Read the model definition and answer for the solid it produces. Units are mm, in the model's axes. A direction names the side the tool comes from. Give positions to 0.01 mm unless a question says otherwise; leave off trailing zeros. Loops run counter-clockwise (first coordinate to the right, second up) from the corner with the lowest first, then second, coordinate; pieces in that order, holes last. Notation, with made-up numbers: (27, 23) -> (50, 23) arc R6 ccw to (50, 27) -> close; hole circle Ø4 at (3.5, -37). An arc over 180 degrees is marked (long way). Return JSON: item names as keys, results as strings. Group by question number.
from build123d import *

# Parameters (mm, degrees)
AUFSATZ_LINEAR_AUSTRAGEN1_DEPTH = 3
SKIZZE2_R                       = 2.05
AUFSATZ_LINEAR_AUSTRAGEN2_DEPTH = 12.5
AUFSATZ_LINEAR_START            = 9.5
AUFSATZ_LINEAR_AUSTRAGEN3_DEPTH = 1.6
SCHNITT_LINEAR_AUSTRAGEN1_REACH = 19.13
SKIZZE4_R                       = 1
FASE1_SIZE                      = 0.4


with BuildPart() as part:
    # Skizze1 → Aufsatz-Linear austragen1 (new body)
    with BuildSketch(Plane.XY):
        with BuildLine():
            Line((2, 0), (2, 5))
            ThreePointArc((2, 5), (0, 7), (-2, 5))
            Line((-2, 5), (-2, 0))
            ThreePointArc((-2, 0), (0, -2), (2, 0))
        make_face()
    extrude(amount=AUFSATZ_LINEAR_AUSTRAGEN1_DEPTH)

    # Skizze2 → Aufsatz-Linear austragen2 (add)
    with BuildSketch(Plane.XY.offset(3)):
        with Locations(Location((0, 0, 0), (0, 0, 167.319616508))):
            Circle(SKIZZE2_R)
    extrude(amount=AUFSATZ_LINEAR_AUSTRAGEN2_DEPTH)

    # Skizze3 → Aufsatz-Linear austragen3 (add)
    with BuildSketch(Plane.XY.offset(3).offset(AUFSATZ_LINEAR_START)):
        with BuildLine():
            Line((-1.25, 3.5), (-1.25, 1.624807681))
            ThreePointArc((-1.25, 1.624807681), (0, 2.05), (1.25, 1.624807681))
            Line((1.25, 1.624807681), (1.25, 3.5))
            ThreePointArc((1.25, 3.5), (0, 4.75), (-1.25, 3.5))
        make_face()
    extrude(amount=AUFSATZ_LINEAR_AUSTRAGEN3_DEPTH)

    # Skizze4 → Schnitt-Linear austragen1 (cut, up to next)
    with BuildSketch(Plane.XY.offset(15.5), mode=Mode.PRIVATE) as schnitt_linear_austragen1_sk1:
        Circle(SKIZZE4_R)
    schnitt_linear_austragen1_tool1 = extrude(schnitt_linear_austragen1_sk1.sketch, amount=-SCHNITT_LINEAR_AUSTRAGEN1_REACH, mode=Mode.PRIVATE) & part.part
    add(schnitt_linear_austragen1_tool1.solids().sort_by_distance((0, 0, 15.5))[0], mode=Mode.SUBTRACT)

    # Fase1
    fase1_edges = [part.edges().sort_by_distance(p)[0] for p in [
        (2, -0.45, 15.5),
    ]]
    chamfer(fase1_edges, length=FASE1_SIZE)


solid = part.part
1. Section A-A on x = 0 is taken. Determine the outline of the cut face in (y, z).
2. Section D-D on z = 13.75 is taken. Determine the outline of the cut face in (x, y), then the cut area to 3 significant figures.
3. Section B-B on y = 2.25 is taken. Determine the outline of the cut face in (x, z), then the cut area to 3 significant figures.
4. Flat-ended cylindrical pins translate along their axes: pin 1 Ø5 at (y, z) = (0.5, 4.5) entering from -X; pin 2 Ø1.5 at (x, z) = (-0.5, 8) entering from +Y; pin 3 Ø1.8 at (y, z) = (2.5, 13.5) entering from -X; pin 4 Ø1.2 at (x, y) = (-0.5, 2.5) entering from +Z. Find the tip coordinate at first contact, or state that the pin passes through.
5. Determine the mould class of faces 1 (the flat face through (1.25, 3, 13)), 2 (the cylindrical face through (0, 7, 1)), 3 (the cylindrical face through (0, -1, 8)), 4 (the cylindrical face through (-0.19, -2.04, 8.97)) for opening direction Y: pulls with the +Y half, pulls with the -Y half, needs draft (parallel to the pull), parting line crosses it, or undercut.
6. Which of the six approach directions +Z, -Z, +X, -X, +Y, -Y give full straight-line access (tool end or side, diameter ignored) to faces 5 (the cylindrical face through (0, -2, 1)), 6 (the flat face through (-1.25, 3, 13)), 7 (the cylindrical face through (0.03, 4.75, 13.29)), 8 (the flat face through (-1, 1, 15.5))?
7. Section C-C on z = 1.25 is taken. Determine the outline of the cut face in (x, y), then the cut area to 3 significant figures.
8. Straight lines are drawn through the part: line 1 (Z direction, x = 0.05, y = 5); line 2 (X direction, y = -0.75, z = 14.75); line 3 (Z direction, x = 0.75, y = 4.25). For each, find the intervals that lie inside material, in ascending order. Write a range as from..to.
Completed:
{
 "1": {"outline": "(-2.05, 3) -> (-2, 3) -> (-2, 0) -> (-1, 0) -> (-1, 15.5) -> (-1.65, 15.5) -> (-2.05, 15.1) -> close; (1, 0) -> (7, 0) -> (7, 3) -> (2.05, 3) -> (2.05, 12.5) -> (4.75, 12.5) -> (4.75, 14.1) -> (2.05, 14.1) -> (2.05, 15.1) -> (1.65, 15.5) -> (1, 15.5) -> close"},
 "2": {"outline": "(-1.25, 1.62) arc R2.05 ccw (long way) to (1.25, 1.62) -> (1.25, 3.5) arc R1.25 ccw to (-1.25, 3.5) -> close; hole circle Ø2 at (0, 0)", "area": "16.5 mm²"},
 "3": {"outline": "(-2, 0) -> (2, 0) -> (2, 3) -> (-2, 3) -> close; (-1.25, 12.5) -> (1.25, 12.5) -> (1.25, 14.1) -> (-1.25, 14.1) -> close", "area": "16.0 mm²"},
 "4": {"pin 1": "stops at x = -2.05", "pin 2": "stops at y = 2.05", "pin 3": "stops at x = -1.28", "pin 4": "stops at z = 15.2"},
 "5": {"face 1": "needs draft", "face 2": "pulls with the +Y half", "face 3": "undercut", "face 4": "parting line crosses it"},
 "6": {"face 5": "-Z, -Y", "face 6": "+Z, -X, +Y", "face 7": "+Z, +Y", "face 8": "+Z, +X, -X, +Y, -Y"},
 "7": {"outline": "(-2, 0) arc R2 ccw to (2, 0) -> (2, 5) arc R2 ccw to (-2, 5) -> close; hole circle Ø2 at (0, 0)", "area": "29.4 mm²"},
 "8": {"line 1": "z = 0..3", "line 2": "x = -1.91..-0.66, 0.66..1.91", "line 3": "z = 0..3, 12.5..14.1"}
}
